For this review, take the finished solid that the model builds, in its own axes (mm). Face numbers are marked on the shaded views. A direction names the side the tool comes from. Round coordinates to 2 decimals unless told otherwise and drop trailing zeros. Write each loop counter-clockwise with the first axis right and the second up, starting at its lowest first coordinate (ties: lowest second). Pieces come first, ordered by that corner, then holes.
from build123d import *

# Parameters (mm, degrees)
BOSS_EXTRUDE1_DEPTH = 24
SKETCH4_W           = 19
SKETCH4_H           = 47.001372255
CUT_EXTRUDE2_DEPTH  = 15
SKETCH6_R           = 1.6
CUT_EXTRUDE4_DEPTH  = 5
CUT_EXTRUDE5_DEPTH  = 2.998627745
FILLET1_R           = 1


with BuildPart() as part:
    # Sketch1 → Boss-Extrude1 (new body)
    with BuildSketch(Plane.XY):
        Polygon((-10, 0), (10, 0), (10, 50), (5, 50), (-10, 3), align=None)
    extrude(amount=BOSS_EXTRUDE1_DEPTH)

    # Sketch4 → Cut-Extrude2 (cut)
    with BuildSketch(Plane.ZY.offset(10)):
        with Locations((12, 26.499313873)):
            Rectangle(SKETCH4_W, SKETCH4_H)
    extrude(amount=-CUT_EXTRUDE2_DEPTH, mode=Mode.SUBTRACT)

    # Sketch6 → Cut-Extrude4 (cut)
    with BuildSketch(Plane(origin=(10, 0, 0), x_dir=(0, 0, -1), z_dir=(1, 0, 0))):
        with Locations((-12, 25)):
            Circle(SKETCH6_R)
        with Locations((-12, 10)):
            Circle(SKETCH6_R)
        with Locations((-12, 40)):
            Circle(SKETCH6_R)
    extrude(amount=-CUT_EXTRUDE4_DEPTH, mode=Mode.SUBTRACT)

    # Sketch7 → Cut-Extrude5 (cut)
    with BuildSketch(Plane(origin=(0, 2.998627745, 0), x_dir=(1, 0, 0), z_dir=(0, 1, 0))):
        with BuildLine():
            Line((-7, -11), (3, -11))
            ThreePointArc((3, -11), (4, -12), (3, -13))
            Line((3, -13), (-7, -13))
            ThreePointArc((-7, -13), (-8, -12), (-7, -11))
        make_face()
    extrude(amount=-CUT_EXTRUDE5_DEPTH, mode=Mode.SUBTRACT)

    # Fillet1
    fillet1_edges = [part.edges().sort_by_distance(p)[0] for p in [
        (5, 2.998627745, 12),
        (-2.5, 2.998627745, 21.5),
        (-2.5, 2.998627745, 2.5),
    ]]
    fillet(fillet1_edges, radius=FILLET1_R - 0.0001)  # a hair under: the kernel refuses the full size


solid = part.part
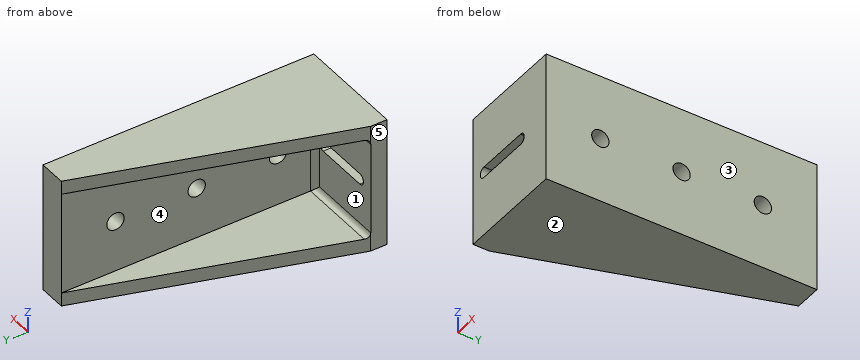
(1) For the marked faces 4 and 5, list the 3-axis set-ups (+Z, -Z, +X, -X, +Y, -Y) from which the entire face can be reached by the end or side of a thin tool; tool diameter is ignored.
Geometry check:
face 4: -X, +Y
face 5: +Z, -Z, -X, +Y, -Y
(2) We need section D-D, the plane x = -5.75. Give the boundary of the cut face in (y, z), and give its area (3 significant figures).
Geometry check:
outline: (0, 0) - (16.32, 0) - (16.32, 2.5) - (4, 2.5) arc R1 cw to (3, 3.5) - (3, 11) - (0, 11) - close; (0, 13) - (3, 13) - (3, 20.5) arc R1 cw to (4, 21.5) - (16.32, 21.5) - (16.32, 24) - (0, 24) - close
area: 133 mm2
(3) Mouldability with a two-part tool opening along Z and no side actions: class the marked faces 1, 2 and 3 as pulls with the +Z half, pulls with the -Z half, needs draft (parallel to the pull), parting line crosses it, or undercut.
Geometry check:
face 1: undercut
face 2: pulls with the -Z half
face 3: needs draft
(4) We need section B-B, the plane z = 19.5. Give the boundary of the cut face in (x, y), and give its area (3 significant figures).
Geometry check:
outline: (-10, 0) - (10, 0) - (10, 50) - (5, 50) - (5, 4) arc R1 cw to (4, 3) - (-10, 3) - close
area: 295 mm2
(5) We need section A-A, the plane y = 25. Give the boundary of the cut face in (x, z), and give its area (3 significant figures).
Geometry check:
outline: (-2.98, 0) - (10, 0) - (10, 10.4) - (5, 10.4) - (5, 2.5) - (-2.98, 2.5) - close; (-2.98, 21.5) - (5, 21.5) - (5, 13.6) - (10, 13.6) - (10, 24) - (-2.98, 24) - close
area: 144 mm2
(6) For pin 1 Ø8 at (y, z) = (19, 20.5) entering from -X; pin 2 Ø5 at (y, z) = (25, 12) entering from -X; pin 3 Ø6 at (y, z) = (29, 5) entering from -X, all flat-tipped, find the tip position at first contact; note any pin that passes through.
Geometry check:
pin 1: stops at x = -6.13
pin 2: stops at x = 5
pin 3: stops at x = -2.23
(7) We need section C-C, the plane x = 5.5. Give the boundary of the cut face in (y, z), and give its area (3 significant figures).
Geometry check:
outline: (0, 0) - (50, 0) - (50, 24) - (0, 24) - close; hole circle Ø3.2 at (10, 12); hole circle Ø3.2 at (25, 12); hole circle Ø3.2 at (40, 12)
area: 1,180 mm2
(8) For line 1 along Y through (x, z) = (8.3, 12); line 2 along Z through (x, y) = (4.25, 45.5); line 3 along X through (y, z) = (20.5, 18.75), list the stretches that pass through material, from the lowest coordinate up.
Geometry check:
line 1: y = 0 to 8.4, 11.6 to 23.4, 26.6 to 38.4, 41.6 to 50
line 2: z = 0 to 2.5, 21.5 to 24
line 3: x = 5 to 10
